Can you work these out from the drawing? Everything is in mm from the part's minimum corner. Coordinates: 2 decimals unless noted, no trailing zeros. Order: outer loops, then holes, each group sorted by start corner. A loop starts at its lowest first (then second) coordinate and runs counter-clockwise, first axis right, second up. Notation, with made-up numbers: (46.5, 0.5) -> (57.5, 0.5) arc R21 cw to (57.5, 33.5) -> close; hole circle Ø3 at (89, -14). An arc over 180 degrees is marked (long way). Return JSON: item names as keys, results as strings. Group by question number.
1) If we section it at D-D, the plane x = 12: Please give me the cut outline in (y, z) (1 decimal).
2) Thinking about a two-plate mould opening in X: for the marked faces 1, 2 and 3, which applies, +X half, -X half, draft (parallel to the pull), parting line (faces both ways), or undercut?
3) If we section it at C-C, the plane y = 2.65: Please give me the cut outline in (x, z), then the cut area to 3 significant figures.
4) If we section it at A-A, the plane x = 38.1: Please give me the cut outline in (y, z) (1 decimal), then the cut area to 3 significant figures.
5) If I drill on probe 1 along Z at (x, y) = (38.1, 3.6); probe 2 along X at (y, z) = (3, 14.5); probe 3 along Z at (x, y) = (15, 3.8) (1 decimal), over which ranges is the centre line in solid material (lowest first)? Write a range as from..to.
6) If we section it at B-B, the plane z = 12.7: Please give me the cut outline in (x, y) (1 decimal), then the cut area to 3 significant figures.
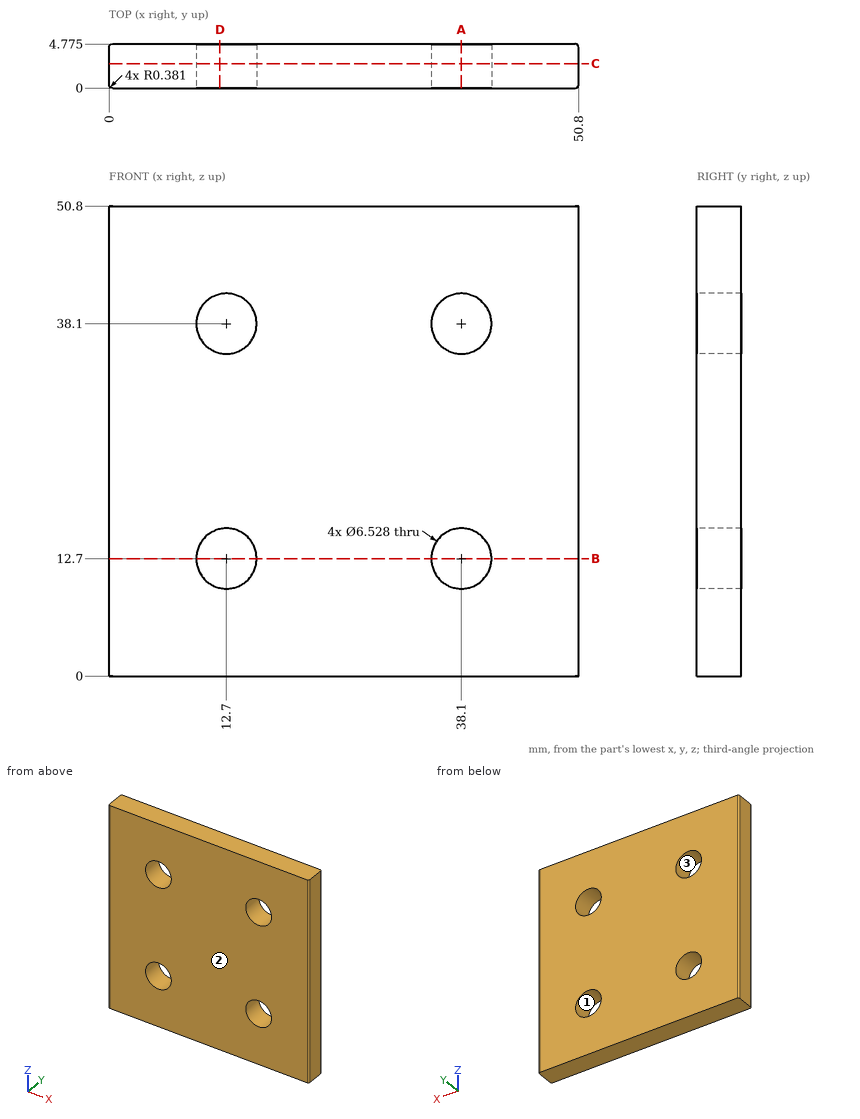
Result sheet:
{
 "1": {"outline": "(0, 0) -> (4.8, 0) -> (4.8, 9.5) -> (0, 9.5) -> close; (0, 15.9) -> (4.8, 15.9) -> (4.8, 34.9) -> (0, 34.9) -> close; (0, 41.3) -> (4.8, 41.3) -> (4.8, 50.8) -> (0, 50.8) -> close"},
 "2": {"face 1": "undercut", "face 2": "draft", "face 3": "undercut"},
 "3": {"outline": "(0, 0) -> (50.8, 0) -> (50.8, 50.8) -> (0, 50.8) -> close; hole circle Ø6.53 at (12.7, 12.7); hole circle Ø6.53 at (12.7, 38.1); hole circle Ø6.53 at (38.1, 12.7); hole circle Ø6.53 at (38.1, 38.1)", "area": "2,450 mm2"},
 "4": {"outline": "(0, 0) -> (4.8, 0) -> (4.8, 9.4) -> (0, 9.4) -> close; (0, 16) -> (4.8, 16) -> (4.8, 34.8) -> (0, 34.8) -> close; (0, 41.4) -> (4.8, 41.4) -> (4.8, 50.8) -> (0, 50.8) -> close", "area": "180 mm2"},
 "5": {"probe 1": "z = 0..9.44, 15.96..34.84, 41.36..50.8", "probe 2": "x = 0..9.98, 15.42..35.38, 40.82..50.8", "probe 3": "z = 0..10.4, 15..35.8, 40.4..50.8"},
 "6": {"outline": "(0, 0.4) arc R0.4 ccw to (0.4, 0) -> (9.4, 0) -> (9.4, 4.8) -> (0.4, 4.8) arc R0.4 ccw to (0, 4.4) -> close; (16, 0) -> (34.8, 0) -> (34.8, 4.8) -> (16, 4.8) -> close; (41.4, 0) -> (50.4, 0) arc R0.4 ccw to (50.8, 0.4) -> (50.8, 4.4) arc R0.4 ccw to (50.4, 4.8) -> (41.4, 4.8) -> close", "area": "180 mm2"}
}
